Autodesk Inventor part; units mm, degrees
ref_plane "YZ Plane" through (0, 0, 0) normal (1, 0, 0) x (0, 1, 0)
ref_plane "XZ Plane" through (0, 0, 0) normal (0, 1, 0) x (-1, 0, 0)
ref_plane "XY Plane" through (0, 0, 0) normal (0, 0, 1) x (1, 0, 0)
sketch "Sketch1" plane through (0, 0, 0) normal (0, 1, 0) x (-1, 0, 0)
  circle A0 centre (0, 0) radius 4.4
  line L0 (9.1763, 0) -> (-11.3805, 0)
  line L1 (0, 0) -> (0, -9.5)
  line L2 (0, -9.5) -> (0, -12)
  line L3 (0, -12) -> (0, -14.74)
  circle A1 centre (0, -9.5) radius 0.7
  circle A2 centre (0, -12) radius 0.7
  circle A3 centre (0, -14.74) radius 0.7
  arc A4 (-2.4994, -15.0614) -> (2.4994, -15.0614) centre (0, -14.74) ccw
  line L4 (2.4994, -15.0614) -> (4.3641, -0.5612)
  line L5 (-2.4994, -15.0614) -> (-4.3641, -0.5612)
  line L6 (0, 0) -> (0, 9.5)
  line L7 (0, 9.5) -> (0, 12)
  line L8 (0, 12) -> (0, 14.74)
  circle A5 centre (0, 9.5) radius 0.7
  circle A6 centre (0, 12) radius 0.7
  circle A7 centre (0, 14.74) radius 0.7
  arc A8 (2.4994, 15.0614) -> (-2.4994, 15.0614) centre (0, 14.74) ccw
  line L9 (2.4994, 15.0614) -> (4.3641, 0.5612)
  line L10 (-2.4994, 15.0614) -> (-4.3641, 0.5612)
  point P0 (4.3641, 0.5612)
  dimension "d0" = 8.8
  dimension "d2" = 9.5
  dimension "d3" = 2.5
  dimension "d4" = 2.74
  dimension "d5" = 1.4
  dimension "d6" = 1.4
  dimension "d7" = 1.4
  dimension "d8" = 5.04
extrude "Extrusion1" add sketch "Sketch1" against normal blind 2 contours A0 L10 A8 L9 | L4 A4 L5 A0
extrude "Extrusion2" add sketch "Sketch1" against normal blind 4 contours L0 L6 A0 | A0 L1 L0 | L1 A0 L0 | L0 A0 L6
sketch "Sketch2" plane through (0, 0, 0) normal (0, 1, 0) x (1, 0, 0)
  circle A0 centre (0, 0) radius 3.785
  circle A1 centre (0, 0) radius 2.75
  dimension "d13" = 7.57
  dimension "d14" = 5.5
extrude "Extrusion3" add sketch "Sketch2" along normal blind 0.45
extrude "Extrusion4" cut sketch "Sketch2" against normal blind 0.58 contours A1
sketch "Sketch3" plane through (0, -4, 0) normal (0, -1, 0) x (1, 0, 0)
  circle A0 centre (0, 0) radius 2.75
  circle A1 centre (0, 0) radius 1.375
  dimension "d19" = 5.5
  dimension "d20" = 2.75
extrude "Extrusion5" cut sketch "Sketch3" against normal through all contours A1
extrude "Extrusion6" cut sketch "Sketch3" against normal blind 3.3
properties part number "MMAE 232 CAD Assignment 2 Servo Horn 6-Nicholas Skiba"
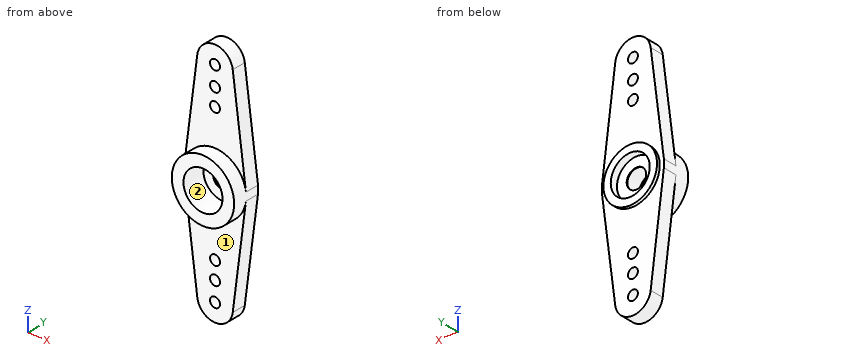
For this review, take the finished solid that the model builds, in its own axes (mm). Face numbers are marked on the shaded views. Coordinates: 2 decimals unless noted, no trailing zeros. Write each loop counter-clockwise with the first axis right and the second up, starting at its lowest first coordinate (ties: lowest second). Pieces come first, ordered by that corner, then holes.
(1) Add section A-A on z = 0. Give the boundary of the cut face in (x, y) (3 decimals).
(2) The part is to be moulded in two halves that separate along Z. For the marked faces 1 and 2, say which applies: +Z half, -Z half, draft (parallel to the pull), parting line (faces both ways), or undercut.
(3) For pin 1 Ø1.6 at (x, z) = (0, 14.74) entering from -Y; pin 2 Ø1.5 at (y, z) = (-1, 12) entering from +X; pin 3 Ø1.5 at (y, z) = (-0.5, 4) entering from -X, all flat-tipped, find the tip position at first contact; note any pin that passes through.
(4) Add section D-D on z = 9.5. Give the boundary of the cut face in (x, y), then the cut area to 3 significant figures.
(5) Add section C-C on x = 0. Count the separate pieces of the cut face and the enclosed holes in it, then the cut area to 3 significant figures.
(6) Add section B-B on y = -2.75. Give the boundary of the cut face in (x, z), then the cut area to 3 significant figures.
(7) Wall thickness on probe 1 along Y at (x, z) = (-3.75, -2.5); probe 2 along Y at (x, z) = (1.75, 4); probe 3 along X at (y, z) = (-0.7, -14.74): over which ranges is each line inside the solid? List them lowest first.
Answer sheet:
1. outline: (-4.4, -4) - (-2.75, -4) - (-2.75, -0.7) - (-1.375, -0.7) - (-1.375, -0.58) - (-2.75, -0.58) - (-2.75, 0.45) - (-3.785, 0.45) - (-3.785, 0) - (-4.4, 0) - close; (1.375, -0.7) - (2.75, -0.7) - (2.75, -4) - (4.4, -4) - (4.4, 0) - (3.785, 0) - (3.785, 0.45) - (2.75, 0.45) - (2.75, -0.58) - (1.375, -0.58) - close
2. face 1: draft
2. face 2: undercut
3. pin 1: stops at y = -2
3. pin 2: stops at x = 2.99
3. pin 3: stops at x = -4.02
4. outline: (-3.21, -2) - (-0.7, -2) - (-0.7, 0) - (-3.21, 0) - close; (0.7, -2) - (3.21, -2) - (3.21, 0) - (0.7, 0) - close
4. area: 10.1 mm2
5. separate pieces: 8
5. enclosed holes: 0
5. area: 49.1 mm2
6. outline: circle Ø8.8 at (0, 0); hole circle Ø5.5 at (0, 0)
6. area: 37.1 mm2
7. probe 1: y = -2 to 0
7. probe 2: y = -4 to 0
7. probe 3: x = -2.54 to -0.7, 0.7 to 2.54
